Geometry check sheet. Reference: the model listing, model coordinates, mm. A direction names the side the tool comes from. Round coordinates to 2 decimals unless told otherwise and drop trailing zeros. Order: outer loops, then holes, each group sorted by start corner. A loop starts at its lowest first (then second) coordinate and runs counter-clockwise, first axis right, second up. Notation, with made-up numbers: (1, -5.75) - (9, -5.75) arc R19 cw to (9, 6.25) - close; hole circle Ø8 at (-11, -3.75). An arc over 180 degrees is marked (long way). One line per question, with ' | ' between items. Start each with the question number.
Q1. Tool access check on faces 1 (the face through (-33, 8, 4.004)), 2 (the face through (26, 8, 0)), 3 (the face through (-66, 9, 9)), 4 (the face through (-33, 8, 2.004)). Record the directions out of +Z, -Z, +X, -X, +Y, -Y that give a thin tool (end or side, any length) a straight path to the whole face; none if there is none.
Q2. Mould release check, pull along X, two halves, no side actions. Record for faces 5 (the face through (25, 8, 6)), 6 (the face through (10.186, 8.112, 2.808)), 7 (the face through (70, 8, 3)): +X half, -X half, draft (parallel to the pull), parting line (faces both ways), or undercut.
Q3. Gauge pin test, flat ends, axial feed: P1, Ø5, axis at x = 37.5, y = 8, coming from the -Z side; P2, Ø5, axis at x = -54, y = 9.5, coming from the +Z side; P3, Ø3.5, axis at x = 58.7, z = 3, coming from the +Y side; P4, Ø5, axis at y = 20.5, z = 0, coming from the +X side. Record the tip position at first contact, or that the pin passes through.
Q4. Sectioned sample at A-A, the plane y = 12.75. Enter the section's corners in (x, z), then the cut area to 3 significant figures.
Q5. Sectioned sample at B-B, the plane z = 7.25. Enter the section's corners in (x, y).
Q6. Sectioned sample at D-D, the plane x = -37. Enter the section's corners in (y, z).
Q7. Material ranges on line 1 along X through (y, z) = (2.25, 2.75); line 2 along X through (y, z) = (15.5, 4.25); line 3 along Z through (x, y) = (27, 15.5), recorded low to high.
Q8. Sectioned sample at C-C, the plane x = 1. Enter the section's corners in (y, z), then the cut area to 3 significant figures.
```python
from build123d import *

# Parameters (mm, degrees)
EXTRUDE_1_DEPTH     = 16
SKETCH_3_R          = 1.5
CUT_EXTRUDE_1_DEPTH = 82.804645345
SKETCH_4_W          = 6
SKETCH_4_H          = 6
EXTRUDE_2_DEPTH     = 16
EXTRUDE_3_DEPTH     = 8


with BuildPart() as part:
    # Эскиз1 → Бобышка-Вытянуть1 (new body)
    with BuildSketch(Plane(origin=(0, 0, 0), x_dir=(1, 0, 0), z_dir=(0, 1, 0))):
        Polygon((0, 0), (-71.525936721, 0), (-71.525936721, 1.396480231), (-71.325936721, 1.396480231), (-71.325936721, 2.8586364), (-75.035652424, 2.8586364), (-80, -0.007531009), (-80, -6), (70, -6), (70, 0), align=None)
    extrude(amount=EXTRUDE_1_DEPTH)

    # Эскиз3 → Вырез-Вытянуть1 (cut, through all)
    with BuildSketch(Plane(origin=(0, 16, 0), x_dir=(1, 0, 0), z_dir=(0, 1, 0))):
        with Locations(Location((8.699103215, -3.003765504, 0), (0, 0, 270))):
            Circle(SKETCH_3_R)
        with Locations(Location((58.699103215, -3.003765504, 0), (0, 0, 270))):
            Circle(SKETCH_3_R)
        Polygon((-47.243192472, 0), (-45.239426968, -2.003765504), (-20.270391363, -2.003765504), (-18.266625858, 0), align=None)
        Polygon((-47.243192472, -6.007531009), (-18.266625858, -6.007531009), (-20.270391363, -4.003765504), (-45.239426968, -4.003765504), align=None)
    extrude(amount=-CUT_EXTRUDE_1_DEPTH, mode=Mode.SUBTRACT)

    # Эскиз4 → Бобышка-Вытянуть2 (add)
    with BuildSketch(Plane.XZ):
        with Locations((-69, 9)):
            Rectangle(SKETCH_4_W, SKETCH_4_H)
    extrude(amount=-EXTRUDE_2_DEPTH)

    # Эскиз5 → Бобышка-Вытянуть3 (add)
    with BuildSketch(Plane(origin=(0, 16, 0), x_dir=(1, 0, 0), z_dir=(0, 1, 0))):
        Polygon((-72, -12), (-72, -6), (-69, -6), (-66, -9), (-66, -12), align=None)
    extrude(amount=EXTRUDE_3_DEPTH)


solid = part.part
```
Determined:
1) face 1: +Z, +Y, -Y | face 2: -Z, +X, +Y, -Y | face 3: +Z, +X, +Y, -Y | face 4: -Z, +Y, -Y
2) face 5: draft | face 6: undercut | face 7: +X half
3) P1: stops at z = 0 | P2: stops at z = 6 | P3: stops at y = 16 | P4: passes through
4) outline: (-80, 0.01) - (-75.04, -2.86) - (-71.33, -2.86) - (-71.33, -1.4) - (-71.53, -1.4) - (-71.53, 0) - (-47.24, 0) - (-45.24, 2) - (-20.27, 2) - (-18.27, 0) - (70, 0) - (70, 6) - (-18.27, 6) - (-20.27, 4) - (-45.24, 4) - (-47.24, 6) - (-66, 6) - (-66, 12) - (-72, 12) - (-72, 6) - (-80, 6) - close; hole circle Ø3 at (8.7, 3); hole circle Ø3 at (58.7, 3) | area: 831 mm2
5) outline: (-72, 0) - (-66, 0) - (-66, 16) - (-67.75, 16) - (-67.75, 24) - (-72, 24) - close
6) outline: (0, 2) - (16, 2) - (16, 4) - (0, 4) - close
7) line 1: x = -80 to 7.22, 10.18 to 57.22, 60.18 to 70 | line 2: x = -80 to -45.49, -20.02 to 7.86, 9.53 to 57.86, 59.53 to 70 | line 3: z = 0 to 6
8) outline: (0, 0) - (16, 0) - (16, 6) - (0, 6) - close | area: 96.0 mm2
